Study the drawing (mm; zero at the part's minimum x, y, z) and answer. Round coordinates to 2 decimals unless told otherwise and drop trailing zeros. Write each loop counter-clockwise with the first axis right and the second up, starting at its lowest first coordinate (ties: lowest second). Pieces come first, ordered by that corner, then holes. Notation, with made-up numbers: M 3,40.25 L 60,40.25 A24 cw 60,61.25 Z; hole C 71,43.5 d7. An arc over 180 degrees is marked long. Write each question's results on one line, items separated by ' | '.
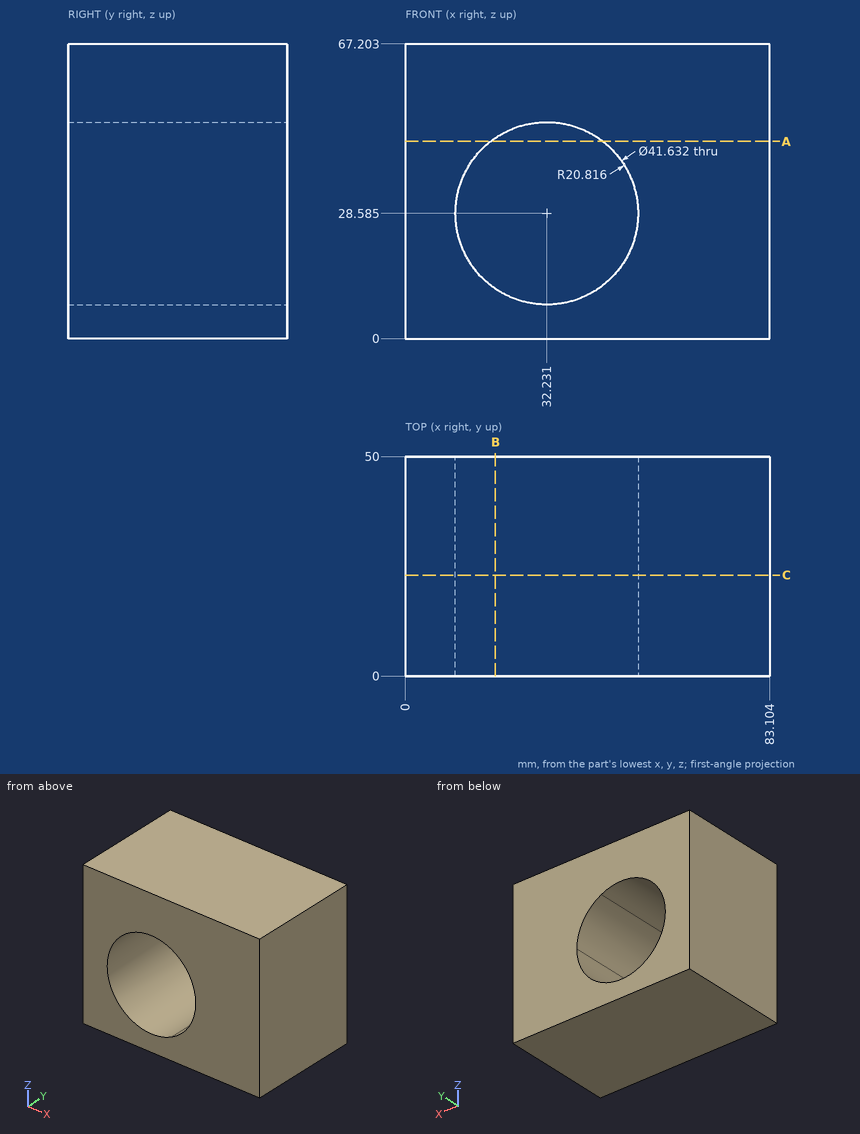
1) Find the intervals of material crossed by line 1 (Z direction, x = 32.5, y = 28); line 2 (X direction, y = 47, z = 37) (1 decimal); line 3 (Z direction, x = 36.5, y = 10), in increasing order.
Return value:
line 1: 0 to 7.77, 49.4 to 67.2 | line 2: 0 to 13.2, 51.3 to 83.1 | line 3: 0 to 8.21, 48.96 to 67.2
2) Section A-A (z = 45) is taken. Determine the outline of the cut face in (x, y), then the cut area to 4 significant figures.
Return value:
outline: M 0,0 L 19.43,0 L 19.43,50 L 0,50 Z; M 45.03,0 L 83.1,0 L 83.1,50 L 45.03,50 Z | area: 2,875 mm²
3) This flat-tipped pin is pushed along its axis until it touches: pin 1 (3 mm diameter, centred on y = 28.5, z = 41, fed in from -X). Where does it stop, or does it pass through?
Return value:
pin 1: x = 0
4) Section C-C (y = 23) is taken. Determine the outline of the cut face in (x, z) (1 decimal).
Return value:
outline: M 0,0 L 83.1,0 L 83.1,67.2 L 0,67.2 Z; hole M 41.6,10 A20.8 ccw 53,28.6 A20.8 ccw 41.6,47.2 A20.8 ccw long Z
5) Section B-B (x = 20.5) is taken. Determine the outline of the cut face in (y, z), then the cut area to 3 significant figures.
Return value:
outline: M 0,0 L 50,0 L 50,11.39 L 0,11.39 Z; M 0,45.78 L 50,45.78 L 50,67.2 L 0,67.2 Z | area: 1,640 mm²
